Input: part model. Units: mm. Frame: model coordinates. A direction names the side the tool comes from. Coordinates: 2 decimals unless noted, no trailing zeros. Order: outer loops, then holes, each group sorted by start corner. A loop starts at its lowest first (then second) coordinate and runs counter-clockwise, first axis right, second up. Notation, with made-up numbers: (2.5, 55) - (36.5, 55) arc R17 cw to (36.5, 67) - close; hole circle Ø6 at (12.25, -10). An arc over 180 degrees is marked (long way). Use a Markdown table: item, result. Add a question column.
Autodesk Fusion 360 part; units mm, degrees
sketch "Base" plane through (0, 0, 0) normal (0, 0, 1) x (1, 0, 0)
  line L0 (0, 0) -> (150, 0)
  line L1 (0, 0) -> (75, -129.9038)
  line L2 (0, 0) -> (150, 0) construction
  line L3 (75, -129.9038) -> (150, 0)
  arc A0 (150, 0) -> (0, 0) centre (75, -290.4738) ccw
  arc A1 (75, -129.9038) -> (150, 0) centre (-139.0576, 80.285) ccw
  arc A2 (0, 0) -> (75, -129.9038) centre (289.0576, 80.285) ccw
  dimension "d1" = 150
  dimension "d3" = 60
  dimension "d4" = 150
  dimension "d5" = 300
  dimension "d7" = 300
  dimension "d8" = 300
extrude "Extrude1" add sketch "Base" along normal blind 4
sketch "Walls" plane through (0, 0, 4) normal (0, 0, 1) x (-1, 0, 0)
  arc A0 (0, 0) -> (-75, 129.9038) centre (-289.0576, -80.285) ccw
  arc A1 (-75, 129.9038) -> (-150, 0) centre (139.0576, -80.285) ccw
  arc A2 (-150, 0) -> (0, 0) centre (-75, 290.4738) ccw
  arc A3 (-75, 124.1541) -> (-145.0206, 2.8749) centre (139.0576, -80.285) ccw
  arc A4 (-145.0206, 2.8749) -> (-4.9794, 2.8749) centre (-75, 290.4738) ccw
  arc A5 (-4.9794, 2.8749) -> (-75, 124.1541) centre (-289.0576, -80.285) ccw
  dimension "d11" = -4
extrude "Extrude2" add sketch "Walls" along normal blind 35
sketch "Cutout" plane through (0, 0, 4) normal (0, 0, 1) x (-1, 0, 0)
  arc A0 (-75, 124.1541) -> (-145.0206, 2.8749) centre (139.0576, -80.285) ccw
  arc A1 (-145.0206, 2.8749) -> (-4.9794, 2.8749) centre (-75, 290.4738) ccw
  arc A2 (-4.9794, 2.8749) -> (-75, 124.1541) centre (-289.0576, -80.285) ccw
  circle A3 centre (-75, 45.1538) radius 47.5
  point P0 (-75, 129.9038)
  dimension "d14" = 95
  dimension "d16" = 84.75
  dimension "d17" = 75
extrude "Extrude3" cut sketch "Cutout" against normal blind 4 contours A3
sketch "Screw holes" plane through (0, 0, 39) normal (0, 0, 1) x (-1, 0, 0)
  arc A0 (-4.9794, 2.8749) -> (-75, 124.1541) centre (-289.0576, -80.285) ccw
  arc A1 (-145.0206, 2.8749) -> (-4.9794, 2.8749) centre (-75, 290.4738) ccw
  arc A2 (-75, 124.1541) -> (-145.0206, 2.8749) centre (139.0576, -80.285) ccw
  arc A3 (-150, 0) -> (0, 0) centre (-75, 290.4738) ccw
  arc A4 (0, 0) -> (-75, 129.9038) centre (-289.0576, -80.285) ccw
  arc A5 (-75, 129.9038) -> (-150, 0) centre (139.0576, -80.285) ccw
  circle A6 centre (-3, 1.5) radius 1
  circle A7 centre (-147, 1.5) radius 1
  circle A8 centre (-75, 126.4038) radius 1
  dimension "d20" = 2
  dimension "d22" = 1.5
  dimension "d23" = 3
  dimension "d24" = 2
  dimension "d25" = 1.5
  dimension "d26" = 3
  dimension "d27" = 2
  dimension "d28" = 3.5
extrude "Extrude4" cut sketch "Screw holes" against normal blind 5 contours A6 | A7 | A8
1) Contact query for flat-ended pins moving along their axis: P1, Ø1, axis at x = 75, y = -126.5, coming from the +Z side; P2, Ø3, axis at x = 92.5, y = -115.5, coming from the +Z side; P3, Ø2, axis at y = -95.5, z = 12.5, coming from the -X side; P4, Ø6, axis at x = 27.5, z = 5.5, coming from the +Y side. Output: stop coordinate, or through.
2) Cut plane B-B (y = -59). Return the cut outline in (x, z), and give its area (3 significant figures).
3) Material intervals for L1, parallel to X at y = -49.5, z = 35; L2, parallel to Y at x = 125.5, z = 19; L3, parallel to X at y = -74, z = 11.5, sorted ascending.
4) Pull-direction query (Y, two-part tool) for faces 3 (the cylindrical face through (117.779, -66.857, 21.255)), 4 (the cylindrical face through (74.01, 5.525, 21.255)), 5 (the cylindrical face through (121.279, -68.795, 19.227)), 6 (the flat face through (75, 7, 39)); classes: pulls with the +Y half, pulls with the -Y half, needs draft (parallel to the pull), parting line crosses it, or undercut.
5) Cut plane C-C (z = 27). Return the cut outline in (x, y), and give its area (3 significant figures).
6) Reachability of faces 1 (the cylindrical face through (29.693, -59.422, 2.028)), 2 (the cylindrical face through (33.21, -68.57, 21.26)) from +Z, -Z, +X, -X, +Y, -Y: full face, straight path, thin tool, end or side. Return the list, or none.
7) Cut plane A-A (x = 115.5). Return the cut outline in (y, z), and give its area (3 significant figures).
8) Cut plane D-D (y = -111.5). Return the cut outline in (x, z).
Computed:
| question | item | result |
|---|---|---|
| 1 | P1 | stops at z = 34 |
| 1 | P2 | passes through |
| 1 | P3 | stops at x = 45.23 |
| 1 | P4 | stops at y = 6.21 |
| 2 | outline | (23.35, 0) - (29.56, 0) - (29.56, 4) - (27.88, 4) - (27.88, 39) - (23.35, 39) - close; (120.44, 0) - (126.65, 0) - (126.65, 39) - (122.12, 39) - (122.12, 4) - (120.44, 4) - close |
| 2 | area | 366 mm2 |
| 3 | L1 | x = 18.58 to 23.03, 126.97 to 131.42 |
| 3 | L2 | y = -61.17 to -52.48, 1.19 to 5.25 |
| 3 | L3 | x = 31.77 to 36.45, 113.55 to 118.23 |
| 4 | face 3 | undercut |
| 4 | face 4 | undercut |
| 4 | face 5 | pulls with the -Y half |
| 4 | face 6 | needs draft |
| 5 | outline | (0, 0) arc R300 ccw to (75, -129.9) arc R300 ccw to (150, 0) arc R300 ccw to start; hole (4.98, -2.87) arc R296 ccw to (75, -124.15) arc R296 ccw to (145.02, -2.87) arc R296 ccw to start |
| 5 | area | 1,760 mm2 |
| 6 | face 1 | +Z, -Z |
| 6 | face 2 | +Z |
| 7 | outline | (-78.46, 0) - (-69.97, 0) - (-69.97, 4) - (-70.77, 4) - (-70.77, 39) - (-78.46, 39) - close; (-20.33, 0) - (6.78, 0) - (6.78, 39) - (2.74, 39) - (2.74, 4) - (-20.33, 4) - close |
| 7 | area | 553 mm2 |
| 8 | outline | (58.37, 0) - (91.63, 0) - (91.63, 39) - (86.41, 39) - (86.41, 4) - (63.59, 4) - (63.59, 39) - (58.37, 39) - close |
